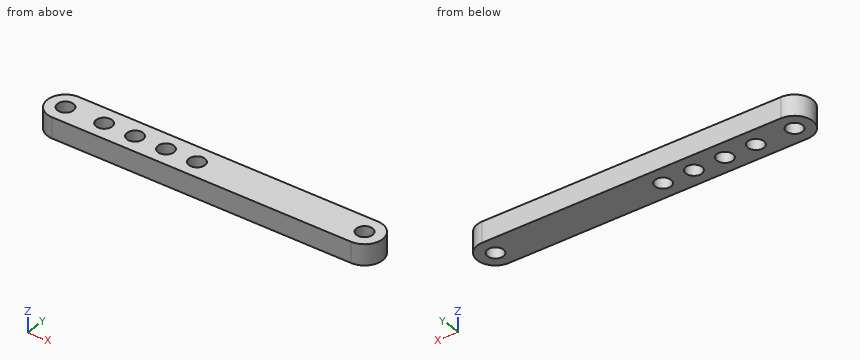
from build123d import *

# Parameters (mm, degrees)
BOSS_EXTRUDE1_DEPTH = 4
SKETCH2_R           = 1.55
CUT_EXTRUDE6_DEPTH  = 38.1913603


with BuildPart() as part:
    # Sketch1 → Boss-Extrude1 (new body)
    with BuildSketch(Plane.XY):
        with BuildLine():
            Line((-33.309608541, 3.5), (24.690391459, 3.5))
            ThreePointArc((24.690391459, 3.5), (28.190391459, 0), (24.690391459, -3.5))
            Line((24.690391459, -3.5), (-33.309608541, -3.5))
            ThreePointArc((-33.309608541, -3.5), (-36.809608541, 0), (-33.309608541, 3.5))
        make_face()
    extrude(amount=BOSS_EXTRUDE1_DEPTH)

    # Sketch2 → Cut-Extrude6 (cut, through all)
    with BuildSketch(Plane.XY):
        with Locations((-33.309608541, 0)):
            Circle(SKETCH2_R)
        with Locations((-19.809608541, 0)):
            Circle(SKETCH2_R)
        with Locations((24.690391459, 0)):
            Circle(SKETCH2_R)
        with Locations((-25.809608541, 0)):
            Circle(SKETCH2_R)
        with Locations((-13.809608541, 0)):
            Circle(SKETCH2_R)
        with Locations((-7.809608541, 0)):
            Circle(SKETCH2_R)
    extrude(amount=CUT_EXTRUDE6_DEPTH, mode=Mode.SUBTRACT)


solid = part.part
Input: part model. Units: mm. Frame: model coordinates. Coordinates: 2 decimals unless noted, no trailing zeros. Order: outer loops, then holes, each group sorted by start corner. A loop starts at its lowest first (then second) coordinate and runs counter-clockwise, first axis right, second up.
1. Cut plane B-B, the plane z = 2.4. Return loops of the section in (x, y).
Checked values:
outline: (-33.31, -3.5) - (24.69, -3.5) arc R3.5 ccw to (24.69, 3.5) - (-33.31, 3.5) arc R3.5 ccw to start; hole circle Ø3.1 at (-33.31, 0); hole circle Ø3.1 at (-25.81, 0); hole circle Ø3.1 at (-19.81, 0); hole circle Ø3.1 at (-13.81, 0); hole circle Ø3.1 at (-7.81, 0); hole circle Ø3.1 at (24.69, 0)
2. Ray query, line 1 along Y through (x, z) = (-26.5, 1.8); line 2 along Y through (x, z) = (-19.5, 1.1); line 3 along X through (y, z) = (-2.75, 0.6). Return the intervals inside material, ascending.
Checked values:
line 1: y = -3.5 to -1.39, 1.39 to 3.5
line 2: y = -3.5 to -1.52, 1.52 to 3.5
line 3: x = -35.47 to 26.86
3. Cut plane A-A, the plane y = 0. Return loops of the section in (x, z).
Checked values:
outline: (-36.81, 0) - (-34.86, 0) - (-34.86, 4) - (-36.81, 4) - close; (-31.76, 0) - (-27.36, 0) - (-27.36, 4) - (-31.76, 4) - close; (-24.26, 0) - (-21.36, 0) - (-21.36, 4) - (-24.26, 4) - close; (-18.26, 0) - (-15.36, 0) - (-15.36, 4) - (-18.26, 4) - close; (-12.26, 0) - (-9.36, 0) - (-9.36, 4) - (-12.26, 4) - close; (-6.26, 0) - (23.14, 0) - (23.14, 4) - (-6.26, 4) - close; (26.24, 0) - (28.19, 0) - (28.19, 4) - (26.24, 4) - close
